Build history of the part. All positions in model axes, mm. A direction names the side the tool comes from. Give positions to 0.01 mm unless a question says otherwise; leave off trailing zeros. Write each loop counter-clockwise with the first axis right and the second up, starting at its lowest first coordinate (ties: lowest second). Pieces come first, ordered by that corner, then holes. Notation, with made-up numbers: (59, 3.25) -> (81, 3.25) arc R18 cw to (81, 38.25) -> close; hole circle Ø10 at (-26, 57.5). An arc over 180 degrees is marked (long way). Put each result on its own line as item: value.
from build123d import *

# Parameters (mm, degrees)
SKETCH1_W               = 5
SKETCH1_H               = 18.37548573
SKETCH1_W_2             = 10
SKETCH1_H_2             = 22
REVOLVE5_ANGLE          = 156
REVOLVE7_ANGLE          = 50
SKETCH4_OUTSIDE_W       = 180.506
SKETCH4_OUTSIDE_H       = 258.157
CUT_EXTRUDE2_DEPTH      = 170
CUT_EXTRUDE3_DEPTH      = 442.672956065
CUT_EXTRUDE3_DEPTH_BACK = 10
SKETCH5_OUTSIDE_W       = 180.506
SKETCH5_OUTSIDE_H       = 258.157


with BuildPart() as part:
    # Sketch1 → Revolve5 (revolve)
    with BuildSketch(Plane.XY):
        with BuildLine():
            Line((560, 85), (150, 85))
            add(Edge.make_bspline(
                [(130, 81.42814839), (131.199611639, 81.653568948), (134.531160345, 82.27353853), (140.063409966, 83.276352633), (145.198462089, 84.177415336), (148.333178957, 84.715838785), (149.39998937, 84.897876633), (149.733326587, 84.954653305), (149.933332963, 84.98866355), (150, 85)],
                knots=[0.892972089, 0.892972089, 0.892972089, 0.892972089, 0.912262482, 0.946527454, 0.981827786, 0.994656092, 0.99679374, 0.998931275, 1, 1, 1, 1], degree=3))
            Line((130, 81.42814839), (130, 78.37548573))
            add(Edge.make_bspline(
                [(130, 78.37548573), (130.416441261, 78.4539748), (131.249429944, 78.610441407), (132.499278387, 78.843638055), (133.749457206, 79.075350404), (134.58311467, 79.228848558), (135, 79.305358628)],
                knots=[0.889993585, 0.889993585, 0.889993585, 0.889993585, 0.896710365, 0.903427144, 0.910143923, 0.916860703, 0.916860703, 0.916860703, 0.916860703], degree=3))
            add(Edge.make_bspline(
                [(135, 79.305358628), (135.41688533, 79.381868697), (140.494804486, 80.310770929), (145.581915204, 81.204990099), (150.253322265, 82)],
                knots=[0.916860703, 0.916860703, 0.916860703, 0.916860703, 0.923577482, 0.99866409, 0.99866409, 0.99866409, 0.99866409], degree=3))
            Line((150.253322265, 82), (545, 82))
            Line((545, 82), (555, 82))
            Line((555, 82), (560, 82))
            Line((560, 82), (560, 85))
        make_face()
        with Locations((132.5, 69.187742865)):
            Rectangle(SKETCH1_W, SKETCH1_H)
        with BuildLine():
            add(Edge.make_bspline(
                [(130, 78.37548573), (130.416441261, 78.4539748), (131.249429944, 78.610441407), (132.499278387, 78.843638055), (133.749457206, 79.075350404), (134.58311467, 79.228848558), (135, 79.305358628)],
                knots=[0.889993585, 0.889993585, 0.889993585, 0.889993585, 0.896710365, 0.903427144, 0.910143923, 0.916860703, 0.916860703, 0.916860703, 0.916860703], degree=3))
            Line((130, 78.37548573), (135, 78.37548573))
            Line((135, 78.37548573), (135, 79.305358628))
        make_face()
        with Locations((550, 71)):
            Rectangle(SKETCH1_W_2, SKETCH1_H_2)
    revolve(axis=Axis((2.999985029, 0, 0), (-1, 0, 0)), revolution_arc=REVOLVE5_ANGLE)

    # Sketch1_9 → Revolve7 (revolve)
    with BuildSketch(Plane.XY):
        with BuildLine():
            Line((130, 78.37548573), (130, 81.42814839))
            add(Edge.make_bspline(
                [(0, 0), (-0.012294225, 3.891554312), (-0.027437579, 8.684958126), (0.361573767, 14.085722357), (0.576098453, 16.090496183), (0.782493435, 17.604822189), (0.986227589, 18.854298664), (1.188670863, 19.931536976), (1.390404268, 20.885679324), (1.591698837, 21.746529091), (1.792703864, 22.533746067), (1.993507167, 23.261083862), (2.253808552, 24.139979457), (2.580573656, 25.146175179), (2.983585386, 26.259501153), (3.385879093, 27.271261727), (3.787683439, 28.201566994), (4.189138614, 29.064817448), (4.590335615, 29.871726974), (5.05331092, 30.74778076), (5.583218589, 31.683457084), (6.185429632, 32.669732492), (6.787226927, 33.590624245), (7.451481511, 34.546094958), (8.182770444, 35.530963646), (8.985083876, 36.540013411), (9.850344603, 37.562485558), (10.782608842, 38.595746542), (11.785011743, 39.636928062), (12.851029789, 40.680352273), (13.983960321, 41.72463117), (15.186170623, 42.768194245), (16.387975322, 43.755294725), (17.654380903, 44.743506811), (18.987602276, 45.731471932), (20.389198856, 46.717890971), (21.790522044, 47.657861765), (23.257103599, 48.59836715), (24.790441056, 49.538186318), (26.391587757, 50.476245251), (28.05829275, 51.412163763), (29.791720393, 52.345056651), (31.59268286, 53.274185034), (33.459445798, 54.199628429), (35.392909821, 55.120726442), (37.459746918, 56.067201212), (39.59327023, 57.006562681), (41.860151348, 57.96659169), (44.193707143, 58.917521836), (46.660609333, 59.885320784), (49.260404933, 60.867669295), (51.99403381, 61.861671206), (54.860992187, 62.865616104), (57.794602823, 63.85555089), (60.861539281, 64.853573463), (64.06149587, 65.858380358), (67.461497598, 66.888166734), (70.995135905, 67.920234745), (74.662088876, 68.953918346), (78.462130407, 69.988575944), (82.462197069, 71.040436012), (86.662284614, 72.107100186), (91.062388571, 73.18640193), (95.662505252, 74.276388609), (100.462631288, 75.375305679), (105.462763855, 76.481579791), (110.662900527, 77.593803027), (116.063039296, 78.710717608), (121.663178505, 79.831201671), (126.331516094, 80.735110576), (129.133123023, 81.265252428), (130, 81.42814839)],
                knots=[0, 0, 0, 0, 0.061462209, 0.075705788, 0.085548437, 0.093321935, 0.099856333, 0.105553797, 0.110642995, 0.115267654, 0.119524592, 0.123482434, 0.127191759, 0.134010181, 0.140199136, 0.145901384, 0.151215493, 0.156212588, 0.160945789, 0.165455878, 0.171870938, 0.177937368, 0.183716425, 0.189254732, 0.196326298, 0.203099892, 0.209625632, 0.217492532, 0.225090541, 0.232464167, 0.24106462, 0.249438142, 0.257620809, 0.265641058, 0.274822876, 0.28384341, 0.292725747, 0.301488561, 0.311376345, 0.321146599, 0.330814589, 0.341584449, 0.352255608, 0.362840299, 0.374512001, 0.386101174, 0.398765505, 0.411352526, 0.425006218, 0.438588433, 0.453231339, 0.468927603, 0.484557057, 0.501237456, 0.517857889, 0.535527769, 0.554243231, 0.574001115, 0.593705628, 0.614453399, 0.636242373, 0.65907093, 0.682937829, 0.707842151, 0.733783254, 0.760760729, 0.78877436, 0.81782409, 0.847909993, 0.879032247, 0.892972089, 0.892972089, 0.892972089, 0.892972089], degree=3))
            Line((0, 0), (2.999985029, 0))
            Line((2.999985029, 0), (2.999985029, 0.009477573))
            add(Edge.make_bspline(
                [(2.999985029, 0.009477573), (2.993793366, 1.969356524), (2.981962234, 5.911210338), (3.144727077, 11.691517384), (3.670861531, 17.326178467), (4.819198941, 22.729714595), (6.752012755, 27.815986079), (10.434016108, 34.068947754), (16.885973109, 40.769818613), (26.31149284, 47.219276633), (36.588463571, 52.532925143), (47.339293153, 57.041613966), (62.05269101, 62.270744564), (80.889819608, 67.717439736), (103.833134388, 73.178156718), (119.843267231, 76.441355647), (128.581608794, 78.107513888), (129.583558739, 78.296996659), (130, 78.37548573)],
                knots=[0, 0, 0, 0, 0.031208253, 0.062416506, 0.093624758, 0.124833011, 0.156041264, 0.187249517, 0.249666023, 0.312082528, 0.374499034, 0.43691554, 0.499332045, 0.624165056, 0.748998068, 0.873831079, 0.883276806, 0.889993585, 0.889993585, 0.889993585, 0.889993585], degree=3))
        make_face()
    revolve(axis=Axis((2.999985029, 0, 0), (1, 0, 0)), revolution_arc=REVOLVE7_ANGLE)


with BuildPart() as revolve7_kept_piece:
    # of the separate pieces the step leaves, the one the design keeps (revolve7_pieces_kept)
    add(part.part.solids().sort_by_distance((560, 85, 0))[0])

    # Sketch4 outside → Cut-Extrude2 (cut)
    with BuildSketch(Plane.ZY.offset(-135)):
        with Locations((-42.5, 3.6745)):
            Rectangle(SKETCH4_OUTSIDE_W, SKETCH4_OUTSIDE_H)
        with BuildLine():
            Line((0, 60), (0, 82.355324155))
            ThreePointArc((0, 82.355324155), (-28.788899936, 77.159566207), (-53.94524406, 62.227888121))
            Line((-53.94524406, 62.227888121), (-10.199695404, 69.941408635))
            ThreePointArc((-10.199695404, 69.941408635), (-8.867471084, 69.008575123), (-9.800304596, 67.676350803))
            Line((-9.800304596, 67.676350803), (-57.112993118, 59.333847287))
            ThreePointArc((-57.112993118, 59.333847287), (-59.561955461, 56.875063765), (-61.905157801, 54.315291165))
            ThreePointArc((-61.905157801, 54.315291165), (-41.293069586, 56.9484186), (-20.5212086, 56.381557247))
            ThreePointArc((-20.5212086, 56.381557247), (-10.41889066, 59.088465181), (0, 60))
        make_face(mode=Mode.SUBTRACT)
    extrude(amount=CUT_EXTRUDE2_DEPTH, mode=Mode.SUBTRACT)

    # Sketch5 outside → Cut-Extrude3 (cut, two sides: drawn at the far end of the back side and taken through both)
    # profile 1 of 2: a face of its own
    with BuildSketch(Plane(origin=(555, 0, 0), x_dir=(0, 0, -1), z_dir=(1, 0, 0)).offset(-CUT_EXTRUDE3_DEPTH_BACK)):
        with Locations((42.5, 3.6745)):
            Rectangle(SKETCH5_OUTSIDE_W, SKETCH5_OUTSIDE_H)
        with BuildLine():
            Line((0, 85), (0, 60))
            ThreePointArc((0, 60), (10.41889066, 59.088465181), (20.5212086, 56.381557247))
            ThreePointArc((20.5212086, 56.381557247), (40.998184687, 56.962818166), (61.326696118, 54.433779432))
            ThreePointArc((61.326696118, 54.433779432), (80.146948816, -17.333972293), (33.352404732, -74.910727527))
            Line((33.352404732, -74.910727527), (34.572614661, -77.6513639))
            ThreePointArc((34.572614661, -77.6513639), (83.142546062, 17.67249372), (0, 85))
        make_face(mode=Mode.SUBTRACT)
    # profile 2 of 2: a face of its own
    with BuildSketch(Plane(origin=(555, 0, 0), x_dir=(0, 0, -1), z_dir=(1, 0, 0)).offset(-CUT_EXTRUDE3_DEPTH_BACK)):
        with BuildLine():
            Line((9.800304596, 67.676350803), (56.482682204, 59.444988107))
            ThreePointArc((56.482682204, 59.444988107), (54.890605033, 60.918153937), (53.260119726, 62.348694026))
            Line((53.260119726, 62.348694026), (10.199695404, 69.941408635))
            ThreePointArc((10.199695404, 69.941408635), (8.867471084, 69.008575123), (9.800304596, 67.676350803))
        make_face()
    extrude(amount=CUT_EXTRUDE3_DEPTH + CUT_EXTRUDE3_DEPTH_BACK, mode=Mode.SUBTRACT)


solid = revolve7_kept_piece.part
1) Tool access for faces 4 (the flat face through (545, 68, -24)), 5 (the flat face through (392, 84, 0)), 6 (the flat face through (555, 68, -24)): list every direction of +Z, -Z, +X, -X, +Y, -Y with a clear straight run to the whole face (end or side of a thin tool).
Filled sheet:
face 4: +Z
face 5: +Z, +X, -X, +Y, -Y
face 6: +Z, +X
2) Pull direction X, two halves, no side cores. Call faces 1 (the flat face through (135, -14.5, -78.3)), 2 (the flat face through (135, 65, -23)), 3 (the flat face through (132.54, 66.03, -32.38)): released by +X, released by -X, zero draft, split by the parting line, or undercut.
Filled sheet:
face 1: released by -X
face 2: undercut
face 3: zero draft
3) Pin check, flat tips, straight feed: pin 1 (4 mm diameter, centred on x = 186, y = -7, fed in from -Z); pin 2 (3 mm diameter, centred on x = 404.5, z = -17.5, fed in from +Y); pin 3 (8 mm diameter, centred on x = 488.5, z = -15.5, fed in from -Y); pin 4 (4.5 mm diameter, centred on y = 60.5, z = -51.5, fed in from -X). Stop position of each tip, or through.
Filled sheet:
pin 1: z = -84.85
pin 2: y = 83.48
pin 3: y = 79.65
pin 4: x = 130
4) Slice it at A-A (x = 412). Write the cut outline in (y, z), plus the area to 3 significant figures.
Filled sheet:
outline: (-77.65, -34.57) arc R85 ccw to (85, 0) -> (82, 0) arc R82 cw to (-74.91, -33.35) -> close
area: 682 mm2
5) Wall check: L1, parallel to X at y = 58, z = -50; L2, parallel to Z at x = 477.5, y = -1; L3, parallel to Y at x = 473.5, z = -48. Give the ranges that are in metal, low to high.
Filled sheet:
L1: 130 to 135, 545 to 555
L2: -84.99 to -81.99
L3: -70.15 to -66.48, 66.48 to 70.15
